Could you check a few things on this model? Use its own coordinates, in mm. Face numbers are marked on the shaded views. A direction names the side the tool comes from. Give positions to 0.01 mm unless a question says otherwise; leave off trailing zeros. Write each loop counter-clockwise with the first axis right and the second up, starting at its lowest first coordinate (ties: lowest second). Pieces come first, ordered by that corner, then holes. Notation, with made-up numbers: M -26.5,55 L 20.5,55 A15 ccw 20.5,71 Z; hole C -13.75,69 d2. An arc over 180 degrees is marked long. Use one line per item in the form item = value.
from build123d import *

# Parameters (mm, degrees)
SKETCH1_W           = 40
SKETCH1_H           = 40
BOSS_EXTRUDE1_DEPTH = 40
SKETCH2_W           = 20
SKETCH2_H           = 20
SKETCH2_W_2         = 10
CUT_EXTRUDE1_DEPTH  = 40
SKETCH3_W           = 20
SKETCH3_H           = 20
CUT_EXTRUDE2_DEPTH  = 40
CUT_EXTRUDE3_DEPTH  = 40
CUT_EXTRUDE4_DEPTH  = 40
CUT_EXTRUDE5_DEPTH  = 10


with BuildPart() as part:
    # Sketch1 → Boss-Extrude1 (new body)
    with BuildSketch(Plane.XY):
        with Locations((20, 20)):
            Rectangle(SKETCH1_W, SKETCH1_H)
    extrude(amount=BOSS_EXTRUDE1_DEPTH)

    # Sketch2 → Cut-Extrude1 (cut)
    with BuildSketch(Plane.XY.offset(40)):
        with Locations((10, 30)):
            Rectangle(SKETCH2_W, SKETCH2_H)
        with Locations((35, 10)):
            Rectangle(SKETCH2_W_2, SKETCH2_H)
    extrude(amount=-CUT_EXTRUDE1_DEPTH, mode=Mode.SUBTRACT)

    # Sketch3 → Cut-Extrude2 (cut)
    with BuildSketch(Plane.ZY.offset(-20)):
        with Locations((30, 30)):
            Rectangle(SKETCH3_W, SKETCH3_H)
    extrude(amount=-CUT_EXTRUDE2_DEPTH, mode=Mode.SUBTRACT)

    # Sketch4 → Cut-Extrude3 (cut)
    with BuildSketch(Plane.ZY.offset(-20)):
        with BuildLine():
            Line((20, 40), (0, 40))
            Line((0, 40), (0, 20))
            ThreePointArc((0, 20), (5.857864376, 34.142135624), (20, 40))
        make_face()
    extrude(amount=-CUT_EXTRUDE3_DEPTH, mode=Mode.SUBTRACT)

    # Sketch5 → Cut-Extrude4 (cut)
    with BuildSketch(Plane.ZY):
        with BuildLine():
            Line((0, 0), (20, 0))
            ThreePointArc((20, 0), (5.857864376, 5.857864376), (0, 20))
            Line((0, 20), (0, 0))
        make_face()
        with BuildLine():
            Line((40, 0), (40, 20))
            ThreePointArc((40, 20), (34.142135624, 5.857864376), (20, 0))
            Line((20, 0), (40, 0))
        make_face()
    extrude(amount=-CUT_EXTRUDE4_DEPTH, mode=Mode.SUBTRACT)

    # Sketch6 → Cut-Extrude5 (cut)
    with BuildSketch(Plane.ZY):
        with BuildLine():
            Line((20, 0), (20, 20))
            Line((20, 20), (40, 20))
            ThreePointArc((40, 20), (34.142135624, 5.857864376), (20, 0))
        make_face()
    extrude(amount=-CUT_EXTRUDE5_DEPTH, mode=Mode.SUBTRACT)


solid = part.part
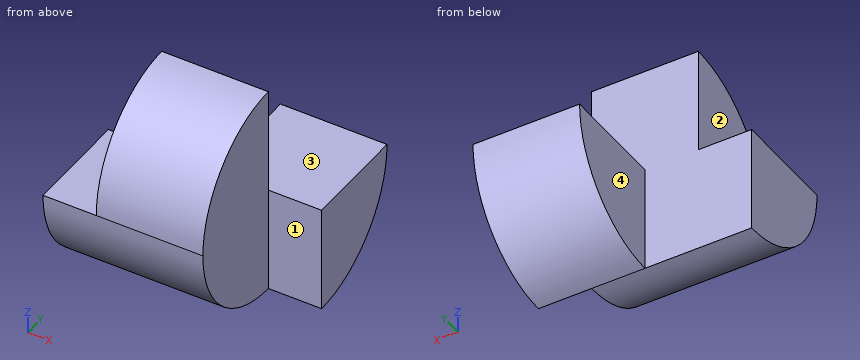
1) I want a section at B-B, the plane z = 10. Please give me the cut outline in (x, y).
Checked values:
outline = M 0,2.68 L 30,2.68 L 30,20 L 40,20 L 40,37.32 L 20,37.32 L 20,20 L 0,20 Z
2) I want a section at D-D, the plane z = 18. Please give me the cut outline in (x, y), plus the area to 3 significant figures.
Checked values:
outline = M 0,0.1 L 30,0.1 L 30,20 L 40,20 L 40,39.9 L 20,39.9 L 20,20 L 0,20 Z
area = 995 mm2
3) For pin 1 Ø16 at (x, y) = (29.5, 29) entering from +Z; pin 2 Ø2 at (x, y) = (9, 7) entering from -Z; pin 3 Ø10 at (y, z) = (12.5, 32) entering from -X; pin 4 Ø3 at (x, y) = (18, 27.5) entering from +Z, each with a flat end and sliding along its axis, tell me the tip position at first contact or that it passes through.
Checked values:
pin_1 = 20
pin_2 = 4
pin_3 = 10
pin_4 = through
4) I want a section at C-C, the plane y = 17. Please give me the cut outline in (x, z).
Checked values:
outline = M 0,0.23 L 30,0.23 L 30,39.77 L 10,39.77 L 10,20 L 0,20 Z
5) If I drill on L1, parallel to X at y = 33.5, z = 12.5; L2, parallel to X at y = 12, z = 21; L3, parallel to Z at x = 29.5, y = 12, over which ranges is the centre line in solid material (lowest first)?
Checked values:
L1 = 20 to 40
L2 = 10 to 30
L3 = 1.67 to 38.33
6) I want a section at A-A, the plane x = 29. Please give me the cut outline in (y, z).
Checked values:
outline = M 20,20 L 20,40 A20 ccw long 40,20 Z
7) For the marked faces 1, 2, 3 and 4, which set-ups out of +Z, -Z, +X, -X, +Y, -Y let a thin tool reach every point of the face, with its end or its side?
Checked values:
face_1 = +Z, -Z, +X, -Y
face_2 = +Z, -X, +Y, -Y
face_3 = +Z, +X, -X, +Y
face_4 = +Z, -Z, -X, +Y
